Could you check a few things on this model? Use its own coordinates, in mm. A direction names the side the tool comes from. Give positions to 0.01 mm unless a question says otherwise; leave off trailing zeros. Loops run counter-clockwise (first coordinate to the right, second up) from the corner with the lowest first, then second, coordinate; pieces in that order, holes last. Notation, with made-up numbers: (15.25, 56) - (20.25, 56) arc R19 ccw to (20.25, 84) - close; hole circle Ø3 at (44, 72.5). An arc over 180 degrees is marked (long way). Write each question's results on one line, items separated by ' | '. Start each with the question number.
```python
from build123d import *

# Parameters (mm, degrees)
SKETCH1_W           = 8.5
SKETCH1_H           = 8.5
BOSS_EXTRUDE1_DEPTH = 3.5
SKETCH2_W           = 8.5
SKETCH2_H           = 8.5
SKETCH2_R           = 1.5
BOSS_EXTRUDE2_DEPTH = 1.5
SKETCH3_W           = 8.5
SKETCH3_H           = 5
BOSS_EXTRUDE3_DEPTH = 3
SKETCH4_W           = 3
SKETCH4_H           = 8.5
BOSS_EXTRUDE4_DEPTH = 6
SKETCH5_W           = 8.5
SKETCH5_H           = 3
BOSS_EXTRUDE5_DEPTH = 27.5
SKETCH6_W           = 3
SKETCH6_H           = 8.5
BOSS_EXTRUDE6_DEPTH = 8
SKETCH7_W           = 8.5
SKETCH7_H           = 5
BOSS_EXTRUDE7_DEPTH = 8.5
CUT_EXTRUDE1_DEPTH  = 3.5
SKETCH10_R          = 1.5
CUT_EXTRUDE3_DEPTH  = 3.5
SKETCH11_W          = 6
SKETCH11_H          = 4.5
CUT_EXTRUDE4_DEPTH  = 3.5
SKETCH12_W          = 4.5
SKETCH12_H          = 6
CUT_EXTRUDE5_DEPTH  = 3.5
SKETCH13_W          = 6
SKETCH13_H          = 4.5
CUT_EXTRUDE6_DEPTH  = 3.5
SKETCH14_W          = 4.5
SKETCH14_H          = 6
CUT_EXTRUDE7_DEPTH  = 3.5


with BuildPart() as part:
    # Sketch1 → Boss-Extrude1 (new body)
    with BuildSketch(Plane(origin=(0, 0, 0), x_dir=(1, 0, 0), z_dir=(0, 1, 0))):
        with Locations((4.25, 4.25)):
            Rectangle(SKETCH1_W, SKETCH1_H)
        Polygon((5.985496764, 7.195964334), (2.575496764, 7.195964334), (0.870496764, 4.242817707), (2.575496764, 1.28967108), (5.985496764, 1.28967108), (7.690496764, 4.242817707), align=None, mode=Mode.SUBTRACT)
    extrude(amount=BOSS_EXTRUDE1_DEPTH)

    # Sketch2 → Boss-Extrude2 (add)
    with BuildSketch(Plane.XZ):
        with Locations((4.25, -4.25)):
            Rectangle(SKETCH2_W, SKETCH2_H)
        with Locations((4.25, -4.25)):
            Circle(SKETCH2_R, mode=Mode.SUBTRACT)
    extrude(amount=BOSS_EXTRUDE2_DEPTH)

    # Sketch3 → Boss-Extrude3 (add)
    with BuildSketch(Plane(origin=(8.5, 0, 0), x_dir=(0, 0, -1), z_dir=(1, 0, 0))):
        with Locations((4.25, 1)):
            Rectangle(SKETCH3_W, SKETCH3_H)
    extrude(amount=BOSS_EXTRUDE3_DEPTH)

    # Sketch4 → Boss-Extrude4 (add)
    with BuildSketch(Plane(origin=(0, 3.5, 0), x_dir=(1, 0, 0), z_dir=(0, 1, 0))):
        with Locations((10, 4.25)):
            Rectangle(SKETCH4_W, SKETCH4_H)
    extrude(amount=BOSS_EXTRUDE4_DEPTH)

    # Sketch5 → Boss-Extrude5 (add)
    with BuildSketch(Plane(origin=(11.5, 0, 0), x_dir=(0, 0, -1), z_dir=(1, 0, 0))):
        with Locations((4.25, 8)):
            Rectangle(SKETCH5_W, SKETCH5_H)
    extrude(amount=BOSS_EXTRUDE5_DEPTH)

    # Sketch6 → Boss-Extrude6 (add)
    with BuildSketch(Plane.XZ.offset(-6.5)):
        with Locations((37.5, -4.25)):
            Rectangle(SKETCH6_W, SKETCH6_H)
    extrude(amount=BOSS_EXTRUDE6_DEPTH)

    # Sketch7 → Boss-Extrude7 (add)
    with BuildSketch(Plane(origin=(39, 0, 0), x_dir=(0, 0, -1), z_dir=(1, 0, 0))):
        with Locations((4.25, 1)):
            Rectangle(SKETCH7_W, SKETCH7_H)
    extrude(amount=BOSS_EXTRUDE7_DEPTH)

    # Sketch8 → Cut-Extrude1 (cut)
    with BuildSketch(Plane(origin=(0, 3.5, 0), x_dir=(1, 0, 0), z_dir=(0, 1, 0))):
        Polygon((46.203146627, 5.955), (43.25, 7.66), (40.296853373, 5.955), (40.296853373, 2.545), (43.25, 0.84), (46.203146627, 2.545), align=None)
    extrude(amount=-CUT_EXTRUDE1_DEPTH, mode=Mode.SUBTRACT)

    # Sketch10 → Cut-Extrude3 (cut)
    with BuildSketch(Plane(origin=(0, 0, 0), x_dir=(1, 0, 0), z_dir=(0, 1, 0))):
        with Locations((43.25, 4.25)):
            Circle(SKETCH10_R)
    extrude(amount=-CUT_EXTRUDE3_DEPTH, mode=Mode.SUBTRACT)

    # Sketch11 → Cut-Extrude4 (cut)
    with BuildSketch(Plane.ZY.offset(-8.5)):
        with Locations((-4.25, 6.5)):
            Rectangle(SKETCH11_W, SKETCH11_H)
    extrude(amount=-CUT_EXTRUDE4_DEPTH, mode=Mode.SUBTRACT)

    # Sketch12 → Cut-Extrude5 (cut)
    with BuildSketch(Plane(origin=(0, 9.5, 0), x_dir=(1, 0, 0), z_dir=(0, 1, 0))):
        with Locations((12.75, 4.25)):
            Rectangle(SKETCH12_W, SKETCH12_H)
    extrude(amount=-CUT_EXTRUDE5_DEPTH, mode=Mode.SUBTRACT)

    # Sketch13 → Cut-Extrude6 (cut)
    with BuildSketch(Plane(origin=(39, 0, 0), x_dir=(0, 0, -1), z_dir=(1, 0, 0))):
        with Locations((4.25, 6.5)):
            Rectangle(SKETCH13_W, SKETCH13_H)
    extrude(amount=-CUT_EXTRUDE6_DEPTH, mode=Mode.SUBTRACT)

    # Sketch14 → Cut-Extrude7 (cut)
    with BuildSketch(Plane(origin=(0, 9.5, 0), x_dir=(1, 0, 0), z_dir=(0, 1, 0))):
        with Locations((34.75, 4.25)):
            Rectangle(SKETCH14_W, SKETCH14_H)
    extrude(amount=-CUT_EXTRUDE7_DEPTH, mode=Mode.SUBTRACT)


solid = part.part
```
Q1. I'm going to push flat-ended pins straight in: pin 1 Ø4 at (y, z) = (6, -7.5) entering from +X; pin 2 Ø1.8 at (y, z) = (6.5, -3.5) entering from +X; pin 3 Ø4.5 at (x, z) = (5.5, -4.5) entering from +Y; pin 4 Ø1 at (x, y) = (35, 1.5) entering from +Z. Where does each tip first touch, or does it pass through?
Q2. I need wall thicknesses on L1, parallel to X at y = 9, z = -5; L2, parallel to Z at x = 4.25, y = -0.4; L3, parallel to X at y = -1, z = -6.75. Which ranges of each line are inside material? Lowest first, please. Write a range as from..to.
Q3. Which directions (+Z, -Z, +X, -X, +Y, -Y) give clear straight access to the entire face, cutting with the end or side of a thin tool? Please do faces 4 (the face through (10, 4.25, -4)), 5 (the face through (36, 2, -4)), 6 (the face through (4, 2, -7.196)), 7 (the face through (8.5, 9, -4)).
Q4. I want a section at B-B, the plane x = 4.25. List the corners of the cut face in (y, z) for me, then the cut area to 3 significant figures.
Q5. If we mould it in two halves opening along Z, with no side actions, what happens to faces 1 (the face through (25, 7, 0)), 2 (the face through (41.794, 1.774, -6.819)), 3 (the face through (39, 9, -4))? For each: +Z half, -Z half, draft (parallel to the pull), parting line (faces both ways), or undercut.
Q6. I want a section at A-A, the plane y = -1. List the corners of the cut face in (x, z) for me, then the cut area to 3 significant figures.
Q7. I want a section at D-D, the plane y = 1.75. State how many separate pieces and enclosed holes the cut face has, then the cut area to 3 significant figures.
Q8. I want a section at C-C, the plane y = 5.5. List the corners of the cut face in (x, z) for me, then the cut area to 3 significant figures.
Conclusion:
1) pin 1: x = 39 | pin 2: x = 32.5 | pin 3: y = 3.5 | pin 4: through
2) L1: 8.5..10.5, 15..32.5, 37..39 | L2: -8.5..-5.75, -2.75..0 | L3: 0..11.5, 36..47.5
3) face 4: +X, -X | face 5: +Z, -Z, -Y | face 6: +Y | face 7: +Z, -Z, -X, +Y
4) outline: (-1.5, -8.5) - (3.5, -8.5) - (3.5, -7.2) - (0, -7.2) - (0, -5.75) - (-1.5, -5.75) - close; (-1.5, -2.75) - (0, -2.75) - (0, -1.29) - (3.5, -1.29) - (3.5, 0) - (-1.5, 0) - close | area: 17.3 mm^2
5) face 1: +Z half | face 2: undercut | face 3: draft
6) outline: (0, -8.5) - (11.5, -8.5) - (11.5, 0) - (0, 0) - close; (36, -8.5) - (47.5, -8.5) - (47.5, 0) - (36, 0) - close; hole circle Ø3 at (4.25, -4.25); hole circle Ø3 at (43.25, -4.25) | area: 181 mm^2
7) separate pieces: 2 | enclosed holes: 2 | area: 135 mm^2
8) outline: (8.5, -8.5) - (11.5, -8.5) - (11.5, -7.25) - (8.5, -7.25) - close; (8.5, -1.25) - (11.5, -1.25) - (11.5, 0) - (8.5, 0) - close; (36, -8.5) - (39, -8.5) - (39, -7.25) - (36, -7.25) - close; (36, -1.25) - (39, -1.25) - (39, 0) - (36, 0) - close | area: 15.0 mm^2
